The listing builds one solid part. Answer for the finished solid, in the listing's coordinates (mm). Round coordinates to 2 decimals unless told otherwise and drop trailing zeros. Write each loop counter-clockwise with the first axis right and the second up, starting at its lowest first coordinate (ties: lowest second). Pieces come first, ordered by that corner, then holes.
Item 1: Find section C-C on x = -68. Give the vertices of the cut face in (y, z).
Item 2: Find section A-A on z = 15. Give the vertices of the cut face in (x, y).
Item 3: Find section B-B on y = -13.5. Give the vertices of the cut face in (x, z).
Item 4: Find the intervals of material crossed by probe 1 along X at (y, z) = (-11.75, -4); probe 2 along Z at (x, y) = (65, -20.25); probe 3 along Z at (x, y) = (-190.5, -5.75), in increasing order.
```python
from build123d import *

# Parameters (mm, degrees)
F0_W     = 450
F0_H     = 250
F0_W_2   = 410
F0_H_2   = 210
F1_DEPTH = 25
F2_R     = 20


with BuildPart() as f1:
    # F0 (on Front) → F1 (new body)
    with BuildSketch(Plane.XZ):
        Rectangle(F0_W, F0_H)
        Rectangle(F0_W_2, F0_H_2, mode=Mode.SUBTRACT)
    extrude(amount=F1_DEPTH)

    # F2
    f2_edges = [f1.edges().sort_by_distance(p)[0] for p in [
        (-205, -12.5, 105),
        (205, -12.5, 105),
        (205, -12.5, -105),
        (-205, -12.5, -105),
        (-225, -12.5, 125),
        (225, -12.5, 125),
        (225, -12.5, -125),
        (-225, -12.5, -125),
    ]]
    fillet(f2_edges, radius=F2_R)


solid = f1.part
```
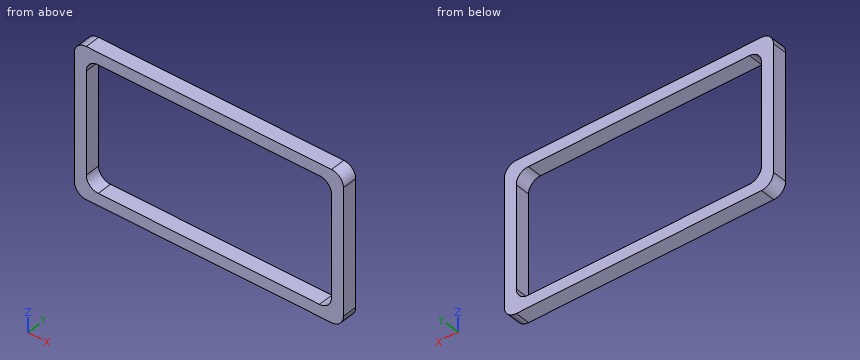
Check values:
1. outline: (-25, -125) - (0, -125) - (0, -105) - (-25, -105) - close; (-25, 105) - (0, 105) - (0, 125) - (-25, 125) - close
2. outline: (-225, -25) - (-205, -25) - (-205, 0) - (-225, 0) - close; (205, -25) - (225, -25) - (225, 0) - (205, 0) - close
3. outline: (-225, -105) arc R20 ccw to (-205, -125) - (205, -125) arc R20 ccw to (225, -105) - (225, 105) arc R20 ccw to (205, 125) - (-205, 125) arc R20 ccw to (-225, 105) - close; hole (-205, -85) arc R20 ccw to (-185, -105) - (185, -105) arc R20 ccw to (205, -85) - (205, 85) arc R20 ccw to (185, 105) - (-185, 105) arc R20 ccw to (-205, 85) - close
4. probe 1: x = -225 to -205, 205 to 225
4. probe 2: z = -125 to -105, 105 to 125
4. probe 3: z = -125 to -104.23, 104.23 to 125
